Source: CAD feature listing. Evaluate the final solid. Frame: model axes, mm. A direction names the side the tool comes from. Give positions to 0.01 mm unless a question says otherwise; leave off trailing zeros. Order: outer loops, then holes, each group sorted by start corner. A loop starts at its lowest first (then second) coordinate and runs counter-clockwise, first axis right, second up.
1) Access query for faces 4 (the face through (3, -1, 0)), 5 (the face through (0, 1.95, 18)). Directions: +Z, -Z, +X, -X, +Y, -Y. A direction counts if a zero-diameter tool reaches every point of the face in a straight line with its end or side. Return the directions, or none.
2) Draft query along X for faces 1 (the face through (3, -1, 35)), 2 (the face through (-6, 0, 17)), 3 (the face through (-0.09, -2.65, 17.26)). Return one class per face: released by +X, released by -X, zero draft, split by the parting line, or undercut.
3) Section B-B, the plane x = 0. Return loops of the section in (y, z), plus the area to 3 significant figures.
4) Section C-C, the plane z = 7. Return loops of the section in (x, y).
5) Material intervals for line 1 (Y direction, x = 0, z = 22); line 2 (Y direction, x = -2.25, z = 18); line 3 (X direction, y = 3, z = 19.5), sorted ascending.
6) Section A-A, the plane y = 0. Return loops of the section in (x, z).
7) First-contact query: P1, Ø3, axis at x = 3, z = 29.5, coming from the -Y side; P2, Ø5, axis at y = -4.5, z = 19.5, coming from the -X side; P3, Ø1.1, axis at x = 1, z = 11, coming from the -Y side; P4, Ø5, axis at x = 0, y = 0, coming from the +Z side. Flat tips, straight axial feed; report the tip coordinate or a pass-through.
```python
from build123d import *

# Parameters (mm, degrees)
SKETCH1_R           = 6
SKETCH1_R_2         = 2.65
BOSS_EXTRUDE1_DEPTH = 35
BOSS_EXTRUDE2_DEPTH = 35
CHAMFER1_SIZE       = 2


with BuildPart() as part:
    # Sketch1 → Boss-Extrude1 (new body)
    with BuildSketch(Plane.XY):
        Circle(SKETCH1_R)
        Circle(SKETCH1_R_2, mode=Mode.SUBTRACT)
    extrude(amount=BOSS_EXTRUDE1_DEPTH)

    # Sketch2 → Boss-Extrude2 (add)
    with BuildSketch(Plane.XY.offset(35)):
        with BuildLine():
            ThreePointArc((1.794435844, 1.95), (0, 2.65), (-1.794435844, 1.95))
            Line((-1.794435844, 1.95), (1.794435844, 1.95))
        make_face()
    extrude(amount=-BOSS_EXTRUDE2_DEPTH)

    # Chamfer1
    chamfer1_edges = [part.edges().sort_by_distance(p)[0] for p in [
        (-6, 0, 0),
        (-6, 0, 35),
    ]]
    chamfer(chamfer1_edges, length=CHAMFER1_SIZE)


solid = part.part
```
From the geometry:
1. face 4: -Z, +X, -X, +Y, -Y
1. face 5: +Z, -Z
2. face 1: zero draft
2. face 2: split by the parting line
2. face 3: undercut
3. outline: (-6, 2) - (-4, 0) - (-2.65, 0) - (-2.65, 35) - (-4, 35) - (-6, 33) - close; (1.95, 0) - (4, 0) - (6, 2) - (6, 33) - (4, 35) - (1.95, 35) - close
3. area: 251 mm2
4. outline: circle Ø12 at (0, 0); hole (-1.79, 1.95) arc R2.65 ccw (long way) to (1.79, 1.95) - close
5. line 1: y = -6 to -2.65, 1.95 to 6
5. line 2: y = -5.56 to -1.4, 1.4 to 5.56
5. line 3: x = -5.2 to 5.2
6. outline: (-6, 2) - (-4, 0) - (-2.65, 0) - (-2.65, 35) - (-4, 35) - (-6, 33) - close; (2.65, 0) - (4, 0) - (6, 2) - (6, 33) - (4, 35) - (2.65, 35) - close
7. P1: stops at y = -5.81
7. P2: stops at x = -5.66
7. P3: stops at y = -5.98
7. P4: stops at z = 35
